Autodesk Inventor part; units mm, degrees
ref_plane "Work Plane1" through (10.95, 0, 0) normal (0, 0, -1) x (1, 0, 0)
ref_plane "YZ Plane" through (0, 0, 0) normal (1, 0, 0) x (0, 1, 0)
ref_plane "XZ Plane" through (0, 0, 0) normal (0, 1, 0) x (-1, 0, 0)
sketch "Sketch1" plane through (0, 0, 0) normal (0, 0, 1) x (1, 0, 0)
  line L0 (-2.52, 0) -> (-2.52, 3.8066)
  line L1 (0, 4.7) -> (0, 2.5)
  line L2 (9, 2.5) -> (25, 2.5)
  line L3 (25, 2.5) -> (25, 0)
  line L4 (25, 0) -> (-2.52, 0)
  arc A0 (0, 4.7) -> (-1.9063, 5.1226) centre (-1, 4.7) ccw
  line L5 (0, -1.1775) -> (0, 7.0651)
  line L6 (-8.024, 0) -> (30.504, 0)
  line L7 (0, 2.5) -> (0.0001, 2.5)
  line L8 (0.0001, 2.5) -> (0.0001, 2.5)
  line L9 (0.0001, 2.5) -> (8.5092, 2.5)
  line L10 (8.5092, 2.5) -> (9, 2.5)
  line L11 (-2.52, 3.8066) -> (-1.9063, 5.1226)
  line L12 (0.0001, 2.5) -> (9, 2.5) construction
  line L13 (9, 2.5) -> (9, 0) construction
  dimension "d0" = 1
  dimension "d1" = 25
  dimension "d2" = 16
  dimension "d3" = 11.4
  dimension "d4" = 5
  dimension "d5" = 2.52
  dimension "d15" = 5
  dimension "d16" = 5
  dimension "d17" = 0.0001
  dimension "d18" = 0.4908
  dimension "d19" = 25
revolve "Body" add sketch "Sketch1" angle 360 about axis through (25, 0, 0) along (-1, 0, 0)
sketch "Sketch2" plane through (0, 0, 0) normal (1, 0, 0) x (0, 0, -1)
  line L0 (3.5, 2.0207) -> (3.5, -2.0207)
  line L1 (3.5, -2.0207) -> (0, -4.0415)
  line L2 (0, -4.0415) -> (-3.5, -2.0207)
  line L3 (-3.5, -2.0207) -> (-3.5, 2.0207)
  line L4 (-3.5, 2.0207) -> (0, 4.0415)
  line L5 (0, 4.0415) -> (3.5, 2.0207)
  point P0 (0, 0)
  point P1 (0, 0)
  dimension "d23" = 7
extrude "Head" add sketch "Sketch2" against normal blind 5.6
sketch "Sketch3" plane through (0, 0, 0) normal (0, 0, 1) x (1, 0, 0)
  line L0 (-5.6, 3.325) -> (-5.6, 4.0415)
  line L1 (-5.6, 4.0415) -> (-5.1864, 4.0415)
  line L2 (-5.1864, 4.0415) -> (-5.6, 3.325)
  line L3 (-6.2379, 0) -> (-1.7726, 0)
  line L4 (-5.6, 4.0415) -> (-5.6, 2.0207)
  line L5 (-2.4105, 4.0415) -> (-5.6, 4.0415)
  point P0 (-5.6, 2.0207)
  dimension "d8" = 30
  dimension "d22" = 6.65
revolve "Chamfer1" cut sketch "Sketch3" angle 360 about axis through (-10, 0, 0) along (1, 0, 0)
thread "Thread"
chamfer "Chamfer2" distance 0.4908 distance2 0.4908 1 edges at (25, -2.5, 0) measured on face at (25, 0.4734, 0.4194)
ref_plane "Work Plane1" through (10.95, 0, 0) normal (0, 0, -1) x (1, 0, 0)
equation "\"d23\" = SW"
equation "\"d6\" = KOH"
equation "\"d10\" = GEL"
equation "\"d13\" = -0.5 * SPD + 0.5 * GD"
equation "\"d14\" = GUL"
equation "\"d0\" = PHH"
equation "\"d1\" = NLG"
equation "\"d2\" = GEL"
equation "\"d3\" = LADI"
equation "\"d4\" = GD"
equation "\"d5\" = 0.45 * KOH"
equation "\"d15\" = SD2"
equation "\"d16\" = BDM"
equation "\"d18\" = GAL"
equation "\"d19\" = KEWI"
equation "\"d8\" = ANG1"
equation "\"d22\" = SW0"
equation "\"NLG\" = 25"
equation "\"GD\" = NND"
equation "\"BDM\" = NND"
equation "\"KOH\" = 5.6"
equation "\"GEL\" = 16"
equation "\"LADI\" = 11.4"
equation "\"SW\" = 7"
equation "\"PHH\" = RR"
equation "\"SW0\" = 6.65"
equation "\"SPD\" = NND - 1.2269 * PTC"
equation "\"SD2\" = NND"
equation "\"SD\" = 0"
equation "\"ANG1\" = 30deg"
equation "\"KEWI\" = 25deg"
equation "\"GAL\" = 0.61345 * PTC"
equation "\"GUL\" = 0.61345 * PTC"
equation "\"PTC\" = 0.8"
equation "\"THREADDIA\" = 5"
equation "\"E0\" = 1.155 * SW"
equation "\"TOA\" = 30deg"
equation "\"NND\" = 5"
equation "\"GD1\" = THREADDIA - 1.2269 * PTC"
equation "\"SDH\" = SW"
equation "\"KOH1\" = 2.3"
equation "\"RR\" = 1"
properties part number "ISO 4162 - M5 x 25" material "Stainless Steel"
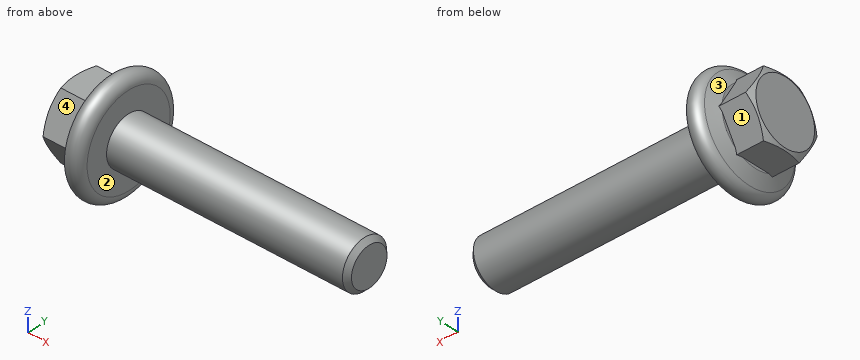
The listing builds one solid part. Answer for the finished solid, in the listing's coordinates (mm). Face numbers are marked on the shaded views. A direction names the side the tool comes from. Give positions to 0.01 mm unless a question says otherwise; leave off trailing zeros. Order: outer loops, then holes, each group sorted by start corner. A loop starts at its lowest first (then second) coordinate and runs counter-clockwise, first axis right, second up. Notation, with made-up numbers: (39, -25) -> (50, -25) arc R34 ccw to (50, 5) -> close; hole circle Ø3 at (-4.75, -31.75). An arc over 180 degrees is marked (long way). Answer as a JSON object with one key per item and string values. Group by question number.
Item 1: Consider L1, parallel to X at y = 1.5, z = -2.25; L2, parallel to Y at x = 8.5, z = 2; L3, parallel to Y at x = 5, z = 0. Determine where each line is inside the solid, lowest interval first. Write a range as from..to.
Item 2: Flat-ended cylindrical pins translate along their axes: pin 1 (2 mm diameter, centred on x = 11.5, z = -4.5, fed in from -Y); pin 2 (6 mm diameter, centred on x = 6.5, y = 3.5, fed in from +Z); pin 3 (3 mm diameter, centred on x = 16, y = -1, fed in from -Z); pin 4 (2 mm diameter, centred on y = 4.5, z = 3.5, fed in from -X). Find the tip coordinate at first contact, or state that the pin passes through.
Item 3: The part is cut by section A-A on y = 0. Write down the section's boundary in (x, z) (3 decimals), and give its area (3 significant figures).
Item 4: The part is cut by section B-B on x = 21.5. Write down the section's boundary in (y, z), and give its area (3 significant figures).
Item 5: A tool of negligible diameter and unlimited length cuts with its end or side. For the marked faces 1, 2, 3 and 4, from which of +Z, -Z, +X, -X, +Y, -Y can it reach the whole face along a straight path? Write none if from no direction.
Result set:
{
 "1": {"L1": "-5.6..0", "L2": "-1.5..1.5", "L3": "-2.5..2.5"},
 "2": {"pin 1": "through", "pin 2": "z = 2.45", "pin 3": "z = -2.5", "pin 4": "x = -2.1"},
 "3": {"outline": "(-5.6, -3.325) -> (-5.499, -3.5) -> (-2.52, -3.5) -> (-2.52, -3.807) -> (-1.906, -5.123) arc R1 ccw to (0, -4.7) -> (0, -2.5) -> (24.509, -2.5) -> (25, -2.009) -> (25, 2.009) -> (24.509, 2.5) -> (0, 2.5) -> (0, 4.7) arc R1 ccw to (-1.906, 5.123) -> (-2.52, 3.807) -> (-2.52, 3.5) -> (-5.499, 3.5) -> (-5.6, 3.325) -> close", "area": "173 mm²"},
 "4": {"outline": "circle Ø5 at (0, 0)", "area": "19.6 mm²"},
 "5": {"face 1": "-Z, -X, +Y", "face 2": "+X", "face 3": "-X", "face 4": "+Z, -X, -Y"}
}
